Part model, mm, in its own coordinate system. Face numbers are marked on the shaded views. A direction names the side the tool comes from. Round coordinates to 2 decimals unless told otherwise and drop trailing zeros. Write each loop counter-clockwise with the first axis right and the second up, starting at its lowest first coordinate (ties: lowest second). Pieces come first, ordered by that corner, then holes. Notation, with made-up numbers: M 51.25,79.25 L 56.25,79.25 A21 ccw 56.25,103.25 Z; hole C 88,-19 d11. An arc over 180 degrees is marked long. Use one line per item in the form item = value. Start each with the question number.
Item 1: Cut at A-A, the plane y = 28. Give the cut face in (x, z), then the cut area to 3 significant figures.
Item 2: Cut at B-B, the plane y = 56.5. Give the cut face in (x, z), then the cut area to 3 significant figures.
Item 3: Probe L1, parallel to X at y = 56.5, z = 14.5; L2, parallel to Z at x = -13, y = 8; L3, parallel to Y at x = 16.6, z = -8.25. List the from-to ranges inside material, lowest first.
Item 4: Mould opens along X. For the marked faces 1, 2, 3 and 4 say: +X half, -X half, draft (parallel to the pull), parting line (faces both ways), or undercut.
Item 5: Flat gauge pins, fed straight in: pin 1 Ø3 at (x, z) = (0, -8) entering from -Y; pin 2 Ø1.6 at (x, y) = (16.5, 16.5) entering from +Z; pin 3 Ø1.6 at (y, z) = (16.5, 19.5) entering from -X; pin 4 Ø2 at (x, y) = (-16.5, 33) entering from -Z. Where does each tip first touch, or does it go through?
Item 6: Which spindle directions (+Z, -Z, +X, -X, +Y, -Y) get a long thin tool onto all of the face, cutting with end or side? Do the marked faces 5 and 6. Say none if no direction does.
from build123d import *

# Parameters (mm, degrees)
SKETCH2_W           = 34.5
SKETCH2_H           = 40.1
BOSS_EXTRUDE1_DEPTH = 2
SKETCH1_R           = 1
SKETCH1_R_2         = 4.25
CUT_EXTRUDE2_DEPTH  = 27.524799716
SKETCH3_W           = 34.5
SKETCH3_H           = 40.1
SKETCH3_W_2         = 30.5
SKETCH3_H_2         = 36.1
BOSS_EXTRUDE3_DEPTH = 160
SKETCH4_W           = 24.336491673
SKETCH4_H           = 45
SKETCH4_H_2         = 40
CUT_EXTRUDE3_DEPTH  = 167.841998609
SKETCH5_W           = 20
SKETCH5_H           = 40
CUT_EXTRUDE4_DEPTH  = 168.778343358
FILLET1_R           = 2.5
SKETCH7_R           = 1.350000001
CUT_EXTRUDE5_DEPTH  = 167.841998609


with BuildPart() as part:
    # Sketch2 → Boss-Extrude1 (new body)
    with BuildSketch(Plane(origin=(0, 0, 0), x_dir=(1, 0, 0), z_dir=(0, 1, 0))):
        Rectangle(SKETCH2_W, SKETCH2_H)
    extrude(amount=BOSS_EXTRUDE1_DEPTH)

    # Sketch1 → Cut-Extrude2 (cut, through all)
    with BuildSketch(Plane(origin=(0, 0, 0), x_dir=(1, 0, 0), z_dir=(0, 1, 0))):
        with Locations(Location((0, 8, 0), (0, 0, 270))):
            Circle(SKETCH1_R)
        with Locations(Location((5.656854249, 5.656854249, 0), (0, 0, 270))):
            Circle(SKETCH1_R)
        with Locations(Location((8, 0, 0), (0, 0, 270))):
            Circle(SKETCH1_R)
        with Locations(Location((5.656854249, -5.656854249, 0), (0, 0, 270))):
            Circle(SKETCH1_R)
        with Locations(Location((0, -8, 0), (0, 0, 270))):
            Circle(SKETCH1_R)
        with Locations(Location((-5.656854249, -5.656854249, 0), (0, 0, 270))):
            Circle(SKETCH1_R)
        with Locations(Location((-8, 0, 0), (0, 0, 270))):
            Circle(SKETCH1_R)
        with Locations(Location((-5.656854249, 5.656854249, 0), (0, 0, 270))):
            Circle(SKETCH1_R)
        with Locations(Location((0, 0, 0), (0, 0, 270))):
            Circle(SKETCH1_R_2)
    extrude(amount=CUT_EXTRUDE2_DEPTH, mode=Mode.SUBTRACT)

    # Sketch3 → Boss-Extrude3 (add)
    with BuildSketch(Plane(origin=(0, 2, 0), x_dir=(1, 0, 0), z_dir=(0, 1, 0))):
        Rectangle(SKETCH3_W, SKETCH3_H)
        Rectangle(SKETCH3_W_2, SKETCH3_H_2, mode=Mode.SUBTRACT)
    extrude(amount=BOSS_EXTRUDE3_DEPTH)

    # Sketch4 → Cut-Extrude3 (cut, through all)
    with BuildSketch(Plane.ZY.offset(17.25)):
        with Locations((0.249999999, 139.5)):
            Rectangle(SKETCH4_W, SKETCH4_H)
        with Locations((0.249999999, 25)):
            Rectangle(SKETCH4_W, SKETCH4_H_2)
    extrude(amount=-CUT_EXTRUDE3_DEPTH, mode=Mode.SUBTRACT)

    # Sketch5 → Cut-Extrude4 (cut, through all)
    with BuildSketch(Plane.XY.offset(20.05)):
        with Locations((0, 25)):
            Rectangle(SKETCH5_W, SKETCH5_H)
        with Locations((0, 137)):
            Rectangle(SKETCH5_W, SKETCH5_H)
    extrude(amount=-CUT_EXTRUDE4_DEPTH, mode=Mode.SUBTRACT)

    # Fillet1
    fillet1_edges = [part.edges().sort_by_distance(p)[0] for p in [
        (16.25, 5, -11.918245837),
        (16.25, 45, -11.918245837),
        (16.25, 45, 12.418245836),
        (16.25, 5, 12.418245836),
        (-16.25, 5, -11.918245837),
        (-16.25, 45, -11.918245837),
        (-16.25, 45, 12.418245836),
        (-16.25, 5, 12.418245836),
        (10, 45, -19.05),
        (10, 5, -19.05),
        (-10, 5, -19.05),
        (-10, 45, -19.05),
        (10, 45, 19.05),
        (10, 5, 19.05),
        (-10, 5, 19.05),
        (-10, 45, 19.05),
        (10, 157, -19.05),
        (10, 117, -19.05),
        (-10, 117, -19.05),
        (-10, 157, -19.05),
        (10, 157, 19.05),
        (10, 117, 19.05),
        (-10, 117, 19.05),
        (-10, 157, 19.05),
        (0, 0, 20.05),
        (-17.25, 0, 0),
        (0, 0, -20.05),
        (15.25, 2, 0),
        (0, 2, -18.05),
        (-15.25, 2, 0),
        (0, 2, 18.05),
        (17.25, 0, 0),
        (17.25, 81, 20.05),
        (-17.25, 81, 20.05),
        (-17.25, 81, -20.05),
        (17.25, 81, -20.05),
        (16.25, 117, 12.418245836),
        (16.25, 117, -11.918245837),
        (-16.25, 117, 12.418245836),
        (-16.25, 117, -11.918245837),
    ]]
    fillet(fillet1_edges, radius=FILLET1_R)

    # Sketch7 → Cut-Extrude5 (cut, through all)
    with BuildSketch(Plane.ZY.offset(17.25)):
        with Locations((-14.750000001, 154.5)):
            Circle(SKETCH7_R)
        with Locations((-14.750000001, 137.5)):
            Circle(SKETCH7_R)
        with Locations((-14.750000001, 120.5)):
            Circle(SKETCH7_R)
        with Locations((15.249999999, 154.5)):
            Circle(SKETCH7_R)
        with Locations((15.249999999, 137.5)):
            Circle(SKETCH7_R)
        with Locations((15.249999999, 120.5)):
            Circle(SKETCH7_R)
        with Locations((-8.250000001, 114.2)):
            Circle(SKETCH7_R)
        with Locations((8.749999999, 114.2)):
            Circle(SKETCH7_R)
    extrude(amount=-CUT_EXTRUDE5_DEPTH, mode=Mode.SUBTRACT)


solid = part.part
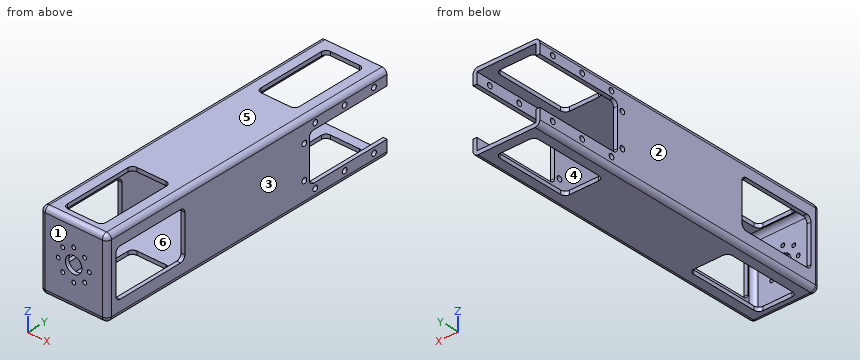
Model answer:
q1.outline = M -17.25,-17.55 A2.5 ccw -14.75,-20.05 L -10,-20.05 L -10,-18.05 L -15.25,-18.05 L -15.25,-11.92 L -17.25,-11.92 Z; M -17.25,12.42 L -15.25,12.42 L -15.25,18.05 L -10,18.05 L -10,20.05 L -14.75,20.05 A2.5 ccw -17.25,17.55 Z; M 10,-20.05 L 14.75,-20.05 A2.5 ccw 17.25,-17.55 L 17.25,-11.92 L 15.25,-11.92 L 15.25,-18.05 L 10,-18.05 Z; M 10,18.05 L 15.25,18.05 L 15.25,12.42 L 17.25,12.42 L 17.25,17.55 A2.5 ccw 14.75,20.05 L 10,20.05 Z
q1.area = 99.7 mm²
q2.outline = M -17.25,-17.55 A2.5 ccw -14.75,-20.05 L 14.75,-20.05 A2.5 ccw 17.25,-17.55 L 17.25,17.55 A2.5 ccw 14.75,20.05 L -14.75,20.05 A2.5 ccw -17.25,17.55 Z; hole M -15.25,-18.05 L 15.25,-18.05 L 15.25,18.05 L -15.25,18.05 Z
q2.area = 277 mm²
q3.L1 = -17.25 to -15.25, 15.25 to 17.25
q3.L2 = -20.05 to -18.05, 18.05 to 20.05
q3.L3 = 0.82 to 5, 45 to 112.85, 115.55 to 117
q4.face_1 = draft
q4.face_2 = -X half
q4.face_3 = +X half
q4.face_4 = undercut
q5.pin_1 = 0
q5.pin_2 = 19.86
q5.pin_3 = -16.97
q5.pin_4 = -19.93
q6.face_5 = +Z, +X, -X, +Y, -Y
q6.face_6 = +Y
